Here's how the part is built. I have some questions about the finished solid (model axes, mm). A direction names the side the tool comes from. Coordinates: 2 decimals unless noted, no trailing zeros. Write each loop counter-clockwise with the first axis right and the second up, starting at its lowest first coordinate (ties: lowest second). Pieces come first, ordered by that corner, then holes.
Item 1: If we mould it in two halves opening along Z, with no side actions, what happens to faces 1 (the face through (-27.15, 26.99, 0.06)), 2 (the face through (19, 15, 4)), 3 (the face through (-20.792, 8.817, -10.736))? For each: pulls with the +Z half, pulls with the -Z half, needs draft (parallel to the pull), parting line crosses it, or undercut.
Item 2: I want a section at C-C (y = 18.75). Please give me the cut outline in (x, z).
Item 3: I want a section at B-B (y = 3.5). Please give me the cut outline in (x, z).
Item 4: I want a section at D-D (x = -23.15). Please give me the cut outline in (y, z).
Item 5: Please list where these lines run through material, in increasing order: line 1 (Z direction, x = 23.15, y = 2); line 2 (X direction, y = 16.5, z = -3); line 3 (Z direction, x = -23.5, y = 9.75).
Item 6: I want a section at A-A (z = 0). Please give me the cut outline in (x, y).
Item 7: For faces 4 (the face through (0, 20, -10)), 5 (the face through (-19, 15, -4)), 6 (the face through (25.49, 8.82, -10.77)), which set-ups out of +Z, -Z, +X, -X, +Y, -Y let a thin tool reach every point of the face, with its end or its side?
Item 8: I'm going to push flat-ended pins straight in: P1, Ø5, axis at x = -6.5, y = 22, coming from the -Z side; P2, Ø2.5, axis at x = -23.5, z = 10, coming from the +Y side; P3, Ø13, axis at x = 20, y = 20, coming from the +Z side; P4, Ø6.5, axis at x = 23.15, z = 9.4, coming from the +Y side. Where does each tip first touch, or does it pass through?
from build123d import *

# Parameters (mm, degrees)
SKETCH2_W           = 60
SKETCH2_H           = 30
BASE_DEPTH          = 10
STRUCTURE_DEPTH     = 20
SKETCH4_R           = 4
ELASTIC_HOLES_DEPTH = 20
SKETCH5_R           = 4.8
PEN_HOLE_DEPTH      = 31
UPPER_CORNER_DEC_R  = 10
BASE_CORNER_DEC_R   = 4
SKETCH6_R           = 2
BOLT_HOLES_DEPTH    = 31
CAP_NUT_HOLES_DEPTH = 2.4


with BuildPart() as part:
    # Sketch2 → Base (new body)
    with BuildSketch(Plane(origin=(0, 0, 0), x_dir=(1, 0, 0), z_dir=(0, 1, 0))):
        Rectangle(SKETCH2_W, SKETCH2_H)
    extrude(amount=BASE_DEPTH)

    # Sketch3 → Structure (add)
    with BuildSketch(Plane(origin=(0, 10, 0), x_dir=(1, 0, 0), z_dir=(0, 1, 0))):
        with BuildLine():
            Line((-9.16515139, 4), (-30, 4))
            Line((-30, 4), (-30, -4))
            Line((-30, -4), (-9.16515139, -4))
            ThreePointArc((-9.16515139, -4), (-10, 0), (-9.16515139, 4))
        make_face()
        with BuildLine():
            ThreePointArc((9.16515139, 4), (0, 10), (-9.16515139, 4))
            Line((-9.16515139, 4), (9.16515139, 4))
        make_face()
        with BuildLine():
            Line((9.16515139, 4), (-9.16515139, 4))
            ThreePointArc((-9.16515139, 4), (-10, 0), (-9.16515139, -4))
            Line((-9.16515139, -4), (9.16515139, -4))
            ThreePointArc((9.16515139, -4), (9.789063129, -2.043096437), (10, 0))
            ThreePointArc((10, 0), (9.789063129, 2.043096437), (9.16515139, 4))
        make_face()
        with BuildLine():
            Line((9.16515139, -4), (-9.16515139, -4))
            ThreePointArc((-9.16515139, -4), (0, -10), (9.16515139, -4))
        make_face()
        with BuildLine():
            Line((30, 4), (9.16515139, 4))
            ThreePointArc((9.16515139, 4), (9.789063129, 2.043096437), (10, 0))
            ThreePointArc((10, 0), (9.789063129, -2.043096437), (9.16515139, -4))
            Line((9.16515139, -4), (30, -4))
            Line((30, -4), (30, 4))
        make_face()
    extrude(amount=STRUCTURE_DEPTH)

    # Sketch4 → Elastic Holes (cut, through all)
    with BuildSketch(Plane.XY.offset(4)):
        with Locations((-20, 20)):
            Circle(SKETCH4_R)
        with Locations((20, 20)):
            Circle(SKETCH4_R)
    extrude(amount=-ELASTIC_HOLES_DEPTH, mode=Mode.SUBTRACT)

    # Sketch5 → Pen Hole (cut, through all)
    with BuildSketch(Plane(origin=(0, 30, 0), x_dir=(1, 0, 0), z_dir=(0, 1, 0))):
        Circle(SKETCH5_R)
    extrude(amount=-PEN_HOLE_DEPTH, mode=Mode.SUBTRACT)

    # Upper Corner Dec
    upper_corner_dec_edges = [part.edges().sort_by_distance(p)[0] for p in [
        (30, 30, 0),
        (-30, 30, 0),
    ]]
    fillet(upper_corner_dec_edges, radius=UPPER_CORNER_DEC_R)

    # Base Corner Dec
    base_corner_dec_edges = [part.edges().sort_by_distance(p)[0] for p in [
        (-30, 5, -15),
        (30, 5, -15),
        (30, 5, 15),
        (-30, 5, 15),
    ]]
    fillet(base_corner_dec_edges, radius=BASE_CORNER_DEC_R)

    # Sketch6 → Bolt Holes (cut, through all)
    with BuildSketch(Plane.XZ):
        with Locations((-23.15, 9.4)):
            Circle(SKETCH6_R)
        with Locations((23.15, 9.4)):
            Circle(SKETCH6_R)
        with Locations((23.15, -9.4)):
            Circle(SKETCH6_R)
        with Locations((-23.15, -9.4)):
            Circle(SKETCH6_R)
    extrude(amount=-BOLT_HOLES_DEPTH, mode=Mode.SUBTRACT)

    # Sketch7 → Cap Nut Holes (cut)
    with BuildSketch(Plane(origin=(0, 10, 0), x_dir=(1, 0, 0), z_dir=(0, 1, 0))):
        Polygon((-21.58538077, 12.11), (-24.71461923, 12.11), (-26.279238459, 9.4), (-24.71461923, 6.69), (-21.58538077, 6.69), (-20.020761541, 9.4), align=None)
        Polygon((20.020761541, 9.4), (21.58538077, 12.11), (24.71461923, 12.11), (26.279238459, 9.4), (24.71461923, 6.69), (21.58538077, 6.69), align=None)
        Polygon((21.58538077, -12.11), (24.71461923, -12.11), (26.279238459, -9.4), (24.71461923, -6.69), (21.58538077, -6.69), (20.020761541, -9.4), align=None)
        Polygon((-20.020761541, -9.4), (-21.58538077, -12.11), (-24.71461923, -12.11), (-26.279238459, -9.4), (-24.71461923, -6.69), (-21.58538077, -6.69), align=None)
    extrude(amount=-CAP_NUT_HOLES_DEPTH, mode=Mode.SUBTRACT)


solid = part.part
Answer:
1. face 1: needs draft
1. face 2: pulls with the +Z half
1. face 3: undercut
2. outline: (-30, -4) - (-23.8, -4) - (-23.8, 4) - (-30, 4) - close; (-16.2, -4) - (-9.17, -4) arc R10 ccw to (9.17, -4) - (16.2, -4) - (16.2, 4) - (9.17, 4) arc R10 ccw to (-9.17, 4) - (-16.2, 4) - close; (23.8, -4) - (30, -4) - (30, 4) - (23.8, 4) - close; hole circle Ø9.6 at (0, 0)
3. outline: (-30, -11) arc R4 ccw to (-26, -15) - (26, -15) arc R4 ccw to (30, -11) - (30, 11) arc R4 ccw to (26, 15) - (-26, 15) arc R4 ccw to (-30, 11) - close; hole circle Ø4 at (-23.15, -9.4); hole circle Ø4 at (-23.15, 9.4); hole circle Ø9.6 at (0, 0); hole circle Ø4 at (23.15, -9.4); hole circle Ø4 at (23.15, 9.4)
4. outline: (0, -15) - (10, -15) - (10, -12.11) - (7.6, -12.11) - (7.6, -11.4) - (0, -11.4) - close; (0, -7.4) - (7.6, -7.4) - (7.6, -6.69) - (10, -6.69) - (10, -4) - (17.53, -4) - (17.53, 4) - (10, 4) - (10, 6.69) - (7.6, 6.69) - (7.6, 7.4) - (0, 7.4) - close; (0, 11.4) - (7.6, 11.4) - (7.6, 12.11) - (10, 12.11) - (10, 15) - (0, 15) - close; (22.47, -4) - (29.49, -4) - (29.49, 4) - (22.47, 4) - close
5. line 1: z = -15 to -11.4, -7.4 to 7.4, 11.4 to 15
5. line 2: x = -30 to -21.94, -18.06 to -3.75, 3.75 to 18.06, 21.94 to 30
5. line 3: z = -15 to -12.11, -6.69 to 6.69, 12.11 to 15
6. outline: (-30, 0) - (-4.8, 0) - (-4.8, 30) - (-20, 30) arc R10 ccw to (-30, 20) - close; (4.8, 0) - (30, 0) - (30, 20) arc R10 ccw to (20, 30) - (4.8, 30) - close; hole circle Ø8 at (-20, 20); hole circle Ø8 at (20, 20)
7. face 4: -Z, +Y
7. face 5: -Z, -X, +Y
7. face 6: +Y
8. P1: stops at z = -9.17
8. P2: passes through
8. P3: stops at z = 4
8. P4: stops at y = 10
